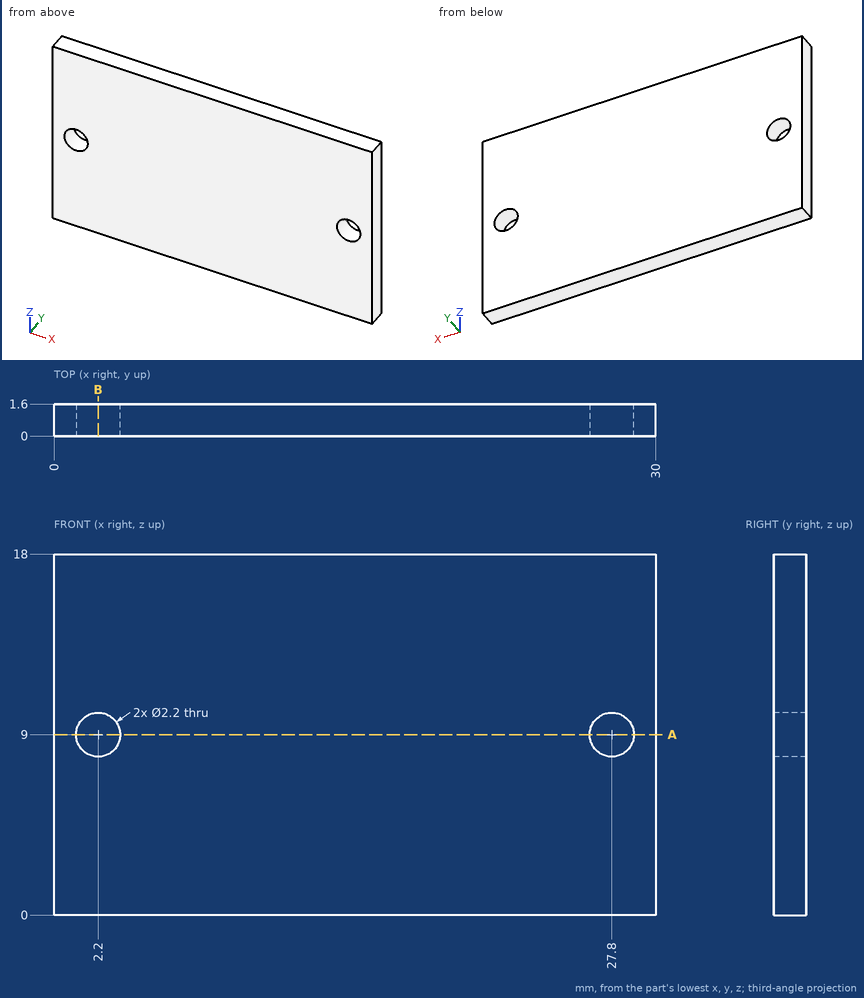
Geometry check sheet. Reference: drawing and pictorial views, mm from the part's lowest x, y, z. Round coordinates to 2 decimals unless told otherwise and drop trailing zeros. Loops run counter-clockwise (first coordinate to the right, second up) from the corner with the lowest first, then second, coordinate; pieces in that order, holes last. Notation, with made-up numbers: M 25.25,-4.75 L 50.25,-4.75 A31 cw 50.25,34.25 Z; hole C 82,16 d11. An arc over 180 degrees is marked long. Return JSON: item names as keys, results as strings. Group by question number.
(1) Scan lines: line 1 along X through (y, z) = (1, 9); line 2 along Z through (x, y) = (27.8, 0.65); line 3 along X through (y, z) = (0.8, 8). Record each from-to range of solid material in increasing order. Write a range as [from, to].
(2) Section check B-B, the plane x = 2.2. Enter the section's corners in (y, z).
(3) Section check A-A, the plane z = 9. Enter the section's corners in (x, y), and give its area (3 significant figures).
Data:
{
 "1": {"line 1": "[0, 1.1], [3.3, 26.7], [28.9, 30]", "line 2": "[0, 7.9], [10.1, 18]", "line 3": "[0, 1.74], [2.66, 27.34], [28.26, 30]"},
 "2": {"outline": "M 0,0 L 1.6,0 L 1.6,7.9 L 0,7.9 Z; M 0,10.1 L 1.6,10.1 L 1.6,18 L 0,18 Z"},
 "3": {"outline": "M 0,0 L 1.1,0 L 1.1,1.6 L 0,1.6 Z; M 3.3,0 L 26.7,0 L 26.7,1.6 L 3.3,1.6 Z; M 28.9,0 L 30,0 L 30,1.6 L 28.9,1.6 Z", "area": "41.0 mm²"}
}
